Build history of the part. All positions in model axes, mm. Round coordinates to 2 decimals unless told otherwise and drop trailing zeros. Write each loop counter-clockwise with the first axis right and the second up, starting at its lowest first coordinate (ties: lowest second). Pieces come first, ordered by that corner, then holes. Notation, with made-up numbers: (28.25, 52.25) - (86.25, 52.25) arc R28 ccw to (86.25, 90.25) - close; hole circle Ø8 at (21.25, 2). An arc over 180 degrees is marked (long way). Answer as a JSON object with one key per item and string values. Group by question number.
Item 1: Probe line 1 (X direction, y = -49, z = 2.3); line 2 (X direction, y = -40.5, z = 3.8); line 3 (Y direction, x = 95, z = 3.7). List the from-to ranges inside material, lowest first. Write a range as from..to.
Item 2: Slice it at C-C, the plane x = 114. List the corners of the cut face in (y, z).
Item 3: Slice it at A-A, the plane x = 98.5. List the corners of the cut face in (y, z), then the cut area to 3 significant figures.
Item 4: Flat gauge pins, fed straight in: pin 1 (0.8 mm diameter, centred on x = 126.5, z = 3.5, fed in from -Y); pin 2 (1 mm diameter, centred on x = 92.33, y = -50.92, fed in from -Z); pin 3 (1.3 mm diameter, centred on x = 110.19, y = -32.59, fed in from +Z); pin 4 (0.5 mm diameter, centred on x = 106.5, z = 3, fed in from -Y). Where does each tip first touch, or does it go through?
Item 5: Slice it at B-B, the plane z = 2.75. Give the number of separate pieces and of enclosed holes in the cut face, then the cut area to 3 significant figures.
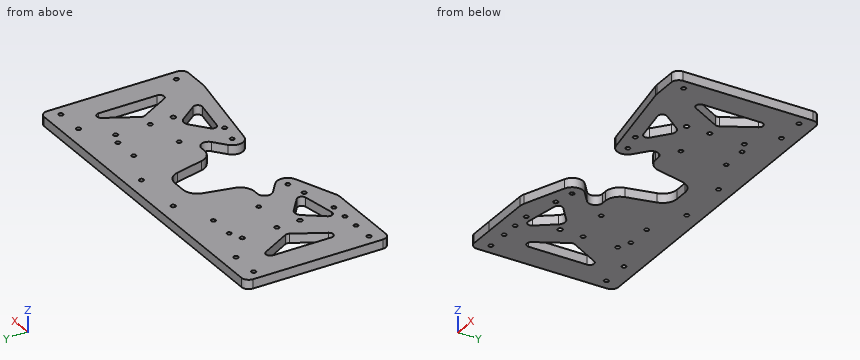
from build123d import *

# Parameters (mm, degrees)
SKETCH1_W           = 233.2
SKETCH1_H           = 100
SKETCH1_R           = 1.55
BOSS_EXTRUDE1_DEPTH = 6.35
FILLET1_R           = 5
SKETCH2_R           = 1.55
CUT_EXTRUDE1_DEPTH  = 6.35
SKETCH3_W           = 10
SKETCH3_H           = 12.7
BOSS_EXTRUDE2_DEPTH = 6.35
FILLET2_R           = 5
FILLET3_R           = 10
FILLET4_R           = 2
FILLET5_R           = 20
FILLET6_R           = 5
CUT_EXTRUDE2_DEPTH  = 10
SKETCH5_W           = 120
SKETCH5_H           = 40
CUT_EXTRUDE4_DEPTH  = 10
SKETCH6_R           = 1.5
CUT_EXTRUDE5_DEPTH  = 10
FILLET7_R           = 10
SKETCH7_W           = 25
SKETCH7_H           = 35
CUT_EXTRUDE6_DEPTH  = 10
FILLET9_R           = 10
SKETCH8_R           = 1.5
CUT_EXTRUDE7_DEPTH  = 10
BOSS_EXTRUDE3_START = -6.35
BOSS_EXTRUDE3_DEPTH = 6.35
FILLET10_R          = 5
BOSS_EXTRUDE4_START = -6.35
BOSS_EXTRUDE4_DEPTH = 6.35
FILLET11_R          = 3
FILLET12_R          = 3
CUT_EXTRUDE8_DEPTH  = 10
FILLET13_R          = 3
CUT_EXTRUDE9_DEPTH  = 10
SKETCH13_R          = 1.55
CUT_EXTRUDE10_DEPTH = 10
SKETCH14_R          = 1.5
CUT_EXTRUDE11_DEPTH = 10
BOSS_EXTRUDE5_START = -6.35
BOSS_EXTRUDE5_DEPTH = 6.35
FILLET14_R          = 10
SKETCH15_R          = 1.55
CUT_EXTRUDE12_DEPTH = 254.816001269
SCALE1_SCALE        = 0.333333333


# Read off the part's stored shape, not the designer's step: Boss-Extrude5
with BuildPart() as part:
    # Sketch1 → Boss-Extrude1 (new body)
    with BuildSketch(Plane.XY):
        with Locations((116.6, -50)):
            Rectangle(SKETCH1_W, SKETCH1_H)
        with Locations((7.5, -10)):
            Circle(SKETCH1_R, mode=Mode.SUBTRACT)
        with Locations((225.7, -10)):
            Circle(SKETCH1_R, mode=Mode.SUBTRACT)
        with Locations((7.5, -90)):
            Circle(SKETCH1_R, mode=Mode.SUBTRACT)
        with Locations((225.7, -90)):
            Circle(SKETCH1_R, mode=Mode.SUBTRACT)
        with Locations((27.5, -10)):
            Circle(SKETCH1_R, mode=Mode.SUBTRACT)
        with Locations((205.7, -10)):
            Circle(SKETCH1_R, mode=Mode.SUBTRACT)
        with Locations((134.6, -10)):
            Circle(SKETCH1_R, mode=Mode.SUBTRACT)
        with Locations((98.6, -10)):
            Circle(SKETCH1_R, mode=Mode.SUBTRACT)
    extrude(amount=BOSS_EXTRUDE1_DEPTH)

    # Fillet1
    fillet1_edges = [part.edges().sort_by_distance(p)[0] for p in [
        (233.2, -100, 3.175),
        (0, -100, 3.175),
        (0, 0, 3.175),
        (233.2, 0, 3.175),
    ]]
    fillet(fillet1_edges, radius=FILLET1_R)

    # Sketch2 → Cut-Extrude1 (cut)
    with BuildSketch(Plane.XY.offset(6.35)):
        with Locations((45, -25)):
            Circle(SKETCH2_R)
        with Locations((45, -49)):
            Circle(SKETCH2_R)
        with Locations(Location((188.2, -49, 0), (0, 0, 180))):
            Circle(SKETCH2_R)
        with Locations(Location((188.2, -25, 0), (0, 0, 180))):
            Circle(SKETCH2_R)
    extrude(amount=-CUT_EXTRUDE1_DEPTH, mode=Mode.SUBTRACT)

    # Sketch3 → Boss-Extrude2 (add)
    with BuildSketch(Plane.XY.offset(6.35)):
        with Locations((125.723568259, 6.35)):
            Rectangle(SKETCH3_W, SKETCH3_H)
        Polygon((120.723568259, 16.7), (120.723568259, 12.7), (130.723568259, 12.7), (130.723568259, 24.7), (85.723568259, 24.7), (85.723568259, 12.7), (95.723568259, 12.7), (95.723568259, 16.7), align=None)
        Polygon((130.723568259, 12.7), (130.723568259, 0), (152.313568259, 0), (130.723568259, 24.7), align=None)
    extrude(amount=-BOSS_EXTRUDE2_DEPTH)

    # Fillet2
    fillet2_edges = [part.edges().sort_by_distance(p)[0] for p in [
        (85.723568259, 12.7, 3.175),
    ]]
    fillet(fillet2_edges, radius=FILLET2_R)

    # Fillet3
    fillet3_edges = [part.edges().sort_by_distance(p)[0] for p in [
        (120.723568259, 0, 3.175),
    ]]
    fillet(fillet3_edges, radius=FILLET3_R)

    # Fillet4
    fillet4_edges = [part.edges().sort_by_distance(p)[0] for p in [
        (85.723568259, 24.7, 3.175),
    ]]
    fillet(fillet4_edges, radius=FILLET4_R)

    # Fillet5
    fillet5_edges = [part.edges().sort_by_distance(p)[0] for p in [
        (130.723568259, 24.7, 3.175),
        (152.313568259, 0, 3.175),
    ]]
    fillet(fillet5_edges, radius=FILLET5_R)

    # Fillet6
    fillet6_edges = [part.edges().sort_by_distance(p)[0] for p in [
        (120.723568259, 16.7, 3.175),
    ]]
    fillet(fillet6_edges, radius=FILLET6_R)

    # Sketch4 → Cut-Extrude2 (cut)
    with BuildSketch(Plane(origin=(0, 0, 0), x_dir=(-1, 0, 0), z_dir=(0, 0, -1))):
        with BuildLine():
            Line((-110.723568259, 0), (-161.395157905, 0))
            ThreePointArc((-161.395157905, 0), (-153.126132222, 1.789475179), (-146.33682816, 6.837678575))
            Line((-146.33682816, 6.837678575), (-136.700308357, 17.862321425))
            ThreePointArc((-136.700308357, 17.862321425), (-129.911004296, 22.910524821), (-121.641978613, 24.7))
            Line((-121.641978613, 24.7), (-87.723568259, 24.7))
            ThreePointArc((-87.723568259, 24.7), (-86.309354696, 24.114213562), (-85.723568259, 22.7))
            Line((-85.723568259, 22.7), (-85.723568259, 17.7))
            ThreePointArc((-85.723568259, 17.7), (-87.188034353, 14.164466094), (-90.723568259, 12.7))
            Line((-90.723568259, 12.7), (-95.723568259, 12.7))
            Line((-95.723568259, 12.7), (-95.723568259, 16.7))
            Line((-95.723568259, 16.7), (-115.723568259, 16.7))
            ThreePointArc((-115.723568259, 16.7), (-119.259102165, 15.235533906), (-120.723568259, 11.7))
            Line((-120.723568259, 11.7), (-120.723568259, 10))
            ThreePointArc((-120.723568259, 10), (-117.794636071, 2.928932188), (-110.723568259, 0))
        make_face()
    extrude(amount=-CUT_EXTRUDE2_DEPTH, mode=Mode.SUBTRACT)

    # Sketch5 → Cut-Extrude4 (cut)
    with BuildSketch(Plane.XY.offset(6.35)):
        Polygon((56.6, -100), (56.6, -60), (26.6, -100), align=None)
        with Locations((116.6, -80)):
            Rectangle(SKETCH5_W, SKETCH5_H)
        Polygon((206.6, -100), (176.6, -60), (176.6, -100), align=None)
    extrude(amount=-CUT_EXTRUDE4_DEPTH, mode=Mode.SUBTRACT)

    # Sketch6 → Cut-Extrude5 (cut)
    with BuildSketch(Plane.XY.offset(6.35)):
        with Locations((71.6, -21.25)):
            Circle(SKETCH6_R)
        with Locations((161.6, -21.25)):
            Circle(SKETCH6_R)
        with Locations((161.6, -52.75)):
            Circle(SKETCH6_R)
        with Locations((71.6, -52.75)):
            Circle(SKETCH6_R)
    extrude(amount=-CUT_EXTRUDE5_DEPTH, mode=Mode.SUBTRACT)

    # Fillet7
    fillet7_edges = [part.edges().sort_by_distance(p)[0] for p in [
        (206.6, -100, 3.175),
        (26.6, -100, 3.175),
        (56.6, -60, 3.175),
        (176.6, -60, 3.175),
    ]]
    fillet(fillet7_edges, radius=FILLET7_R)

    # Sketch7 → Cut-Extrude6 (cut)
    with BuildSketch(Plane.XY.offset(6.35)):
        Polygon((96.1, -60), (104.1, -60), (104.1, -25), align=None)
        Polygon((129.1, -25), (129.1, -60), (137.1, -60), align=None)
        with Locations((116.6, -42.5)):
            Rectangle(SKETCH7_W, SKETCH7_H)
    extrude(amount=-CUT_EXTRUDE6_DEPTH, mode=Mode.SUBTRACT)

    # Fillet9
    fillet9_edges = [part.edges().sort_by_distance(p)[0] for p in [
        (137.1, -60, 3.175),
        (96.1, -60, 3.175),
        (104.1, -25, 3.175),
        (129.1, -25, 3.175),
    ]]
    fillet(fillet9_edges, radius=FILLET9_R)

    # Sketch8 → Cut-Extrude7 (cut)
    with BuildSketch(Plane.XY.offset(6.35)):
        with Locations((53.6, -21.25)):
            Circle(SKETCH8_R)
    extrude(amount=-CUT_EXTRUDE7_DEPTH, mode=Mode.SUBTRACT)

    # Sketch9 → Boss-Extrude3 (add)
    with BuildSketch(Plane.XY.offset(6.35).offset(BOSS_EXTRUDE3_START)):
        with BuildLine():
            Line((53.6, -64), (52.97582451, -64.832233986))
            Line((52.97582451, -64.832233986), (80.428117061, -87.022837132))
            ThreePointArc((80.428117061, -87.022837132), (90.975638571, -85.904897064), (89.857698503, -75.357375554))
            Line((89.857698503, -75.357375554), (70.858883385, -60))
            Line((70.858883385, -60), (61.6, -60))
            ThreePointArc((61.6, -60), (57.127864045, -61.05572809), (53.6, -64))
        make_face()
        with BuildLine():
            ThreePointArc((83.976361625, -80.247148199), (85.642998156, -79.775924736), (86.642907782, -81.190106343))
            ThreePointArc((86.642907782, -81.190106343), (84.642817409, -82.60428795), (83.976361625, -80.247148199))
        make_face(mode=Mode.SUBTRACT)
    boss_extrude3 = extrude(amount=BOSS_EXTRUDE3_DEPTH)

    # Mirror1: Boss-Extrude3 across plane
    add(boss_extrude3.mirror(Plane.ZY.offset(-116.6)))

    # Fillet10
    fillet10_edges = [part.edges().sort_by_distance(p)[0] for p in [
        (52.97582451, -64.832233986, 3.175),
        (70.858883385, -60, 3.175),
        (180.22417549, -64.832233986, 3.175),
        (162.341116615, -60, 3.175),
    ]]
    fillet(fillet10_edges, radius=FILLET10_R)

    # Sketch10 → Boss-Extrude4 (add)
    with BuildSketch(Plane.XY.offset(6.35).offset(BOSS_EXTRUDE4_START)):
        with BuildLine():
            ThreePointArc((29.6, -96), (26.844092638, -98.514663376), (23.358283237, -99.844208453))
            Line((23.358283237, -99.844208453), (86.46162021, -88.573262682))
            ThreePointArc((86.46162021, -88.573262682), (83.276282006, -88.454107183), (80.428117061, -87.022837132))
            Line((80.428117061, -87.022837132), (72.798322589, -80.855419933))
            Line((72.798322589, -80.855419933), (36.033483436, -87.422022085))
            Line((36.033483436, -87.422022085), (29.6, -96))
        make_face()
    boss_extrude4 = extrude(amount=BOSS_EXTRUDE4_DEPTH)

    # Fillet11
    fillet11_edges = [part.edges().sort_by_distance(p)[0] for p in [
        (36.033483436, -87.422022085, 3.175),
        (72.798322589, -80.855419933, 3.175),
    ]]
    fillet(fillet11_edges, radius=FILLET11_R)

    # Mirror3: Boss-Extrude4 across plane
    add(boss_extrude4.mirror(Plane.ZY.offset(-116.6)))

    # Fillet12
    fillet12_edges = [part.edges().sort_by_distance(p)[0] for p in [
        (197.166516564, -87.422022085, 3.175),
        (160.401677411, -80.855419933, 3.175),
    ]]
    fillet(fillet12_edges, radius=FILLET12_R)

    # Sketch11 → Cut-Extrude8 (cut)
    with BuildSketch(Plane.XY.offset(6.35)):
        Polygon((35.5, -50), (18, -82), (18, -18), align=None)
        Polygon((215.2, -18), (215.2, -82), (197.7, -50), align=None)
    extrude(amount=-CUT_EXTRUDE8_DEPTH, mode=Mode.SUBTRACT)

    # Fillet13
    fillet13_edges = [part.edges().sort_by_distance(p)[0] for p in [
        (35.5, -50, 3.175),
        (18, -82, 3.175),
        (18, -18, 3.175),
        (215.2, -18, 3.175),
        (215.2, -82, 3.175),
        (197.7, -50, 3.175),
    ]]
    fillet(fillet13_edges, radius=FILLET13_R)

    # Sketch12 → Cut-Extrude9 (cut)
    with BuildSketch(Plane.XY.offset(6.35)):
        with BuildLine():
            ThreePointArc((186.5, -65), (188.2, -66.7), (189.9, -65))
            ThreePointArc((189.9, -65), (188.2, -63.3), (186.5, -65))
        make_face()
        with BuildLine():
            ThreePointArc((43.3, -65), (45, -66.7), (46.7, -65))
            ThreePointArc((46.7, -65), (45, -63.3), (43.3, -65))
        make_face()
    extrude(amount=-CUT_EXTRUDE9_DEPTH, mode=Mode.SUBTRACT)

    # Sketch13 → Cut-Extrude10 (cut)
    with BuildSketch(Plane.XY.offset(6.35)):
        with Locations((161.599999999, -84.25)):
            Circle(SKETCH13_R)
        with Locations((71.6, -84.25)):
            Circle(SKETCH13_R)
    extrude(amount=-CUT_EXTRUDE10_DEPTH, mode=Mode.SUBTRACT)

    # Sketch14 → Cut-Extrude11 (cut)
    with BuildSketch(Plane(origin=(0, 0, 0), x_dir=(-1, 0, 0), z_dir=(0, 0, -1))):
        with Locations((-22.5, -90)):
            Circle(SKETCH14_R)
        with Locations((-35, -90)):
            Circle(SKETCH14_R)
        with Locations((-47.5, -90)):
            Circle(SKETCH14_R)
    extrude(amount=-CUT_EXTRUDE11_DEPTH, mode=Mode.SUBTRACT)

    # Boss-Extrude5 outline → Boss-Extrude5 (add)
    with BuildSketch(Plane(origin=(0, 0, 0), x_dir=(-1, 0, 0), z_dir=(0, 0, -1)).offset(BOSS_EXTRUDE5_START)):
        with BuildLine():
            Line((-87.900343264, -88.164814191), (-58.358283237, -99.844208453))
            Line((-58.358283237, -99.844208453), (-21.684763887, -99.999640748))
            ThreePointArc((-21.684763887, -99.999640748), (-22.524794828, -99.957145902), (-23.358283237, -99.844208453))
            Line((-23.358283237, -99.844208453), (-86.46162021, -88.573262682))
            ThreePointArc((-86.46162021, -88.573262682), (-87.191188278, -88.404990057), (-87.900343264, -88.164814191))
        make_face()
    extrude(amount=BOSS_EXTRUDE5_DEPTH)

    # Fillet14
    fillet14_edges = [part.edges().sort_by_distance(p)[0] for p in [
        (58.358283237, -99.844208453, 3.175),
    ]]
    fillet(fillet14_edges, radius=FILLET14_R)

    # Sketch15 → Cut-Extrude12 (cut, through all)
    with BuildSketch(Plane(origin=(0, 0, 0), x_dir=(-1, 0, 0), z_dir=(0, 0, -1))):
        with Locations((-179.6, -21.25)):
            Circle(SKETCH15_R)
    extrude(amount=-CUT_EXTRUDE12_DEPTH, mode=Mode.SUBTRACT)


with BuildPart() as part_1:
    # Scale1: scaled about (115.992000253, -43.884971814, 3.175)
    add(part.part.scale(SCALE1_SCALE).moved(Location((77.328000169, -29.256647876, 2.116666667))))


solid = part_1.part
Geometry says:
{
 "1": {"line 1": "x = 77.33..83.33, 87.48..107.99, 124.4..144.91, 149.06..155.06", "line 2": "x = 77.33..83.33, 86.2..111.36, 121.03..146.19, 149.06..155.06", "line 3": "y = -62.55..-57.39, -51.61..-36.8, -35.88..-29.26"},
 "2": {"outline": "(-37.66, 2.12) - (-29.26, 2.12) - (-29.26, 4.23) - (-37.66, 4.23) - close"},
 "3": {"outline": "(-61.86, 2.12) - (-56.76, 2.12) - (-56.76, 4.23) - (-61.86, 4.23) - close; (-53.71, 2.12) - (-29.26, 2.12) - (-29.26, 4.23) - (-53.71, 4.23) - close", "area": "62.5 mm^2"},
 "4": {"pin 1": "stops at y = -58.9", "pin 2": "passes through", "pin 3": "stops at z = 4.23", "pin 4": "stops at y = -58.79"},
 "5": {"separate pieces": "1", "enclosed holes": "31", "area": "1,930 mm^2"}
}
